Source: three-view drawing plus pictorial views. Frame: mm from the lowest corner of the part. A direction names the side the tool comes from. Round coordinates to 2 decimals unless told otherwise and drop trailing zeros. Order: outer loops, then holes, each group sorted by start corner. A loop starts at its lowest first (then second) coordinate and runs counter-clockwise, first axis right, second up. Notation, with made-up numbers: (2, 49.5) -> (19, 49.5) arc R27 ccw to (19, 79.5) -> close; hole circle Ø4 at (62, 73). An arc over 180 degrees is marked (long way). Use a Markdown table: item, result.
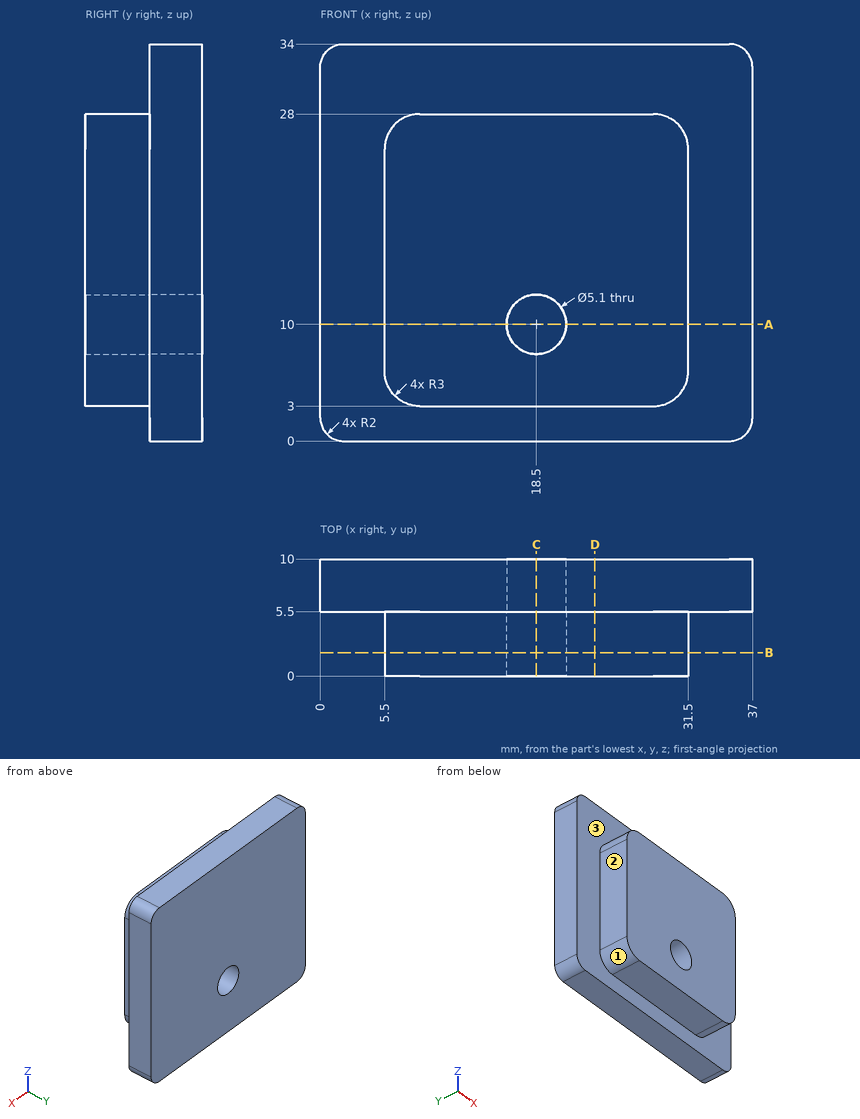
1) Cut plane B-B on y = 2. Return loops of the section in (x, z), and give its area (3 significant figures).
Results found:
| item | result |
|---|---|
| outline | (5.5, 6) arc R3 ccw to (8.5, 3) -> (28.5, 3) arc R3 ccw to (31.5, 6) -> (31.5, 25) arc R3 ccw to (28.5, 28) -> (8.5, 28) arc R3 ccw to (5.5, 25) -> close; hole circle Ø5.1 at (18.5, 10) |
| area | 622 mm² |
2) Line query: L1, parallel to X at y = 1.15, z = 10; L2, parallel to Z at x = 18.5, y = 7; L3, parallel to Y at x = 5, z = 9. Output: solid intervals per line, ascending. Write a range as [from, to].
Results found:
| item | result |
|---|---|
| L1 | x = [5.5, 15.95], [21.05, 31.5] |
| L2 | z = [0, 7.45], [12.55, 34] |
| L3 | y = [5.5, 10] |
3) Cut plane D-D on x = 23.5. Return loops of the section in (y, z), and give its area (4 significant figures).
Results found:
| item | result |
|---|---|
| outline | (0, 3) -> (5.5, 3) -> (5.5, 0) -> (10, 0) -> (10, 34) -> (5.5, 34) -> (5.5, 28) -> (0, 28) -> close |
| area | 290.5 mm² |
4) Set-up query: the marked faces 1, 2 and 3. Return all of +Z, -Z, +X, -X, +Y, -Y with unobstructed straight access to the full face (end or side cutting, diameter ignored); none if empty.
Results found:
| item | result |
|---|---|
| face 1 | -Z, -X, -Y |
| face 2 | +Z, -Z, -X, -Y |
| face 3 | -Y |
5) Pin query (flat end, axial travel): pin 1 Ø4.5 at (x, y) = (15, 2.5) entering from +Z; pin 2 Ø1.6 at (y, z) = (3, 17.5) entering from -X; pin 3 Ø5 at (x, z) = (4, 29.5) entering from -Y. Return the tip coordinate at first contact, or that it passes through.
Results found:
| item | result |
|---|---|
| pin 1 | stops at z = 28 |
| pin 2 | stops at x = 5.5 |
| pin 3 | stops at y = 5.5 |
6) Cut plane C-C on x = 18.5. Return loops of the section in (y, z).
Results found:
| item | result |
|---|---|
| outline | (0, 3) -> (5.5, 3) -> (5.5, 0) -> (10, 0) -> (10, 7.45) -> (0, 7.45) -> close; (0, 12.55) -> (10, 12.55) -> (10, 34) -> (5.5, 34) -> (5.5, 28) -> (0, 28) -> close |
7) Cut plane A-A on z = 10. Return loops of the section in (x, y).
Results found:
| item | result |
|---|---|
| outline | (0, 5.5) -> (5.5, 5.5) -> (5.5, 0) -> (15.95, 0) -> (15.95, 10) -> (0, 10) -> close; (21.05, 0) -> (31.5, 0) -> (31.5, 5.5) -> (37, 5.5) -> (37, 10) -> (21.05, 10) -> close |
